from build123d import *

# Parameters (mm, degrees)
SKETCH1_W           = 6
SKETCH1_H           = 4
BOSS_EXTRUDE1_DEPTH = 3


with BuildPart() as part:
    # Sketch1 → Boss-Extrude1 (new body)
    with BuildSketch(Plane.XY):
        Polygon((0, 29.9), (5, 29.9), (5, 32.9), (20.8, 32.9), (20.8, 29.9), (33, 29.9), (33, 32.9), (48.8, 32.9), (48.8, 29.9), (53.8, 29.9), (53.8, 22.85), (56.9, 22.85), (56.9, 7.05), (53.8, 7.05), (53.8, 0), (48.8, 0), (48.8, -3.1), (33, -3.1), (33, 0), (20.8, 0), (20.8, -3.1), (5, -3.1), (5, 0), (0, 0), (0, 7.05), (-3.1, 7.05), (-3.1, 22.85), (0, 22.85), align=None)
        with Locations((33.8, 12)):
            Rectangle(SKETCH1_W, SKETCH1_H, mode=Mode.SUBTRACT)
    extrude(amount=BOSS_EXTRUDE1_DEPTH)


solid = part.part
Geometry check sheet. Reference: the model listing, model coordinates, mm. A direction names the side the tool comes from. Give positions to 0.01 mm unless a question says otherwise; leave off trailing zeros. Write each loop counter-clockwise with the first axis right and the second up, starting at its lowest first coordinate (ties: lowest second). Pieces come first, ordered by that corner, then holes.
1) Release check for a two-part mould opening along Y. For faces 6 (the face through (-2, 7.05, 1)), 7 (the face through (33, 31, 1)), 8 (the face through (-2, 22.85, 1)), 9 (the face through (30.8, 12, 1)) record: released by +Y, released by -Y, zero draft, split by the parting line, or undercut.
Values follow:
face 6: released by -Y
face 7: zero draft
face 8: released by +Y
face 9: undercut
2) Cross-section at D-D (x = 29.5). Record the boundary of the cut face in (y, z).
Values follow:
outline: (0, 0) - (29.9, 0) - (29.9, 3) - (0, 3) - close
3) Thickness scan on line 1 (X direction, y = 27, z = 1); line 2 (Y direction, x = 25.5, z = 2.45). Record the ranges inside material, lowest first.
Values follow:
line 1: x = 0 to 53.8
line 2: y = 0 to 29.9
4) Go/stop test with flat-tipped pins: pin 1 Ø0.9 at (y, z) = (26.5, 1) entering from +X; pin 2 Ø1.5 at (x, z) = (51, 1.5) entering from -Y; pin 3 Ø0.9 at (x, z) = (56, 2) entering from +Y; pin 4 Ø1 at (x, y) = (11, 9) entering from -Z. Record where each tip stops, or that it passes through.
Values follow:
pin 1: stops at x = 53.8
pin 2: stops at y = 0
pin 3: stops at y = 22.85
pin 4: stops at z = 0
5) Cross-section at A-A (y = 12). Record the boundary of the cut face in (x, z), plus the area to 3 significant figures.
Values follow:
outline: (-3.1, 0) - (30.8, 0) - (30.8, 3) - (-3.1, 3) - close; (36.8, 0) - (56.9, 0) - (56.9, 3) - (36.8, 3) - close
area: 162 mm2
6) Set-up check for faces 1 (the face through (5, 31, 1)), 2 (the face through (20.8, 31, 1)), 3 (the face through (51, 29.9, 1)), 4 (the face through (53.8, 4, 1)), 5 (the face through (5, -2, 1)): record each of +Z, -Z, +X, -X, +Y, -Y from which the full face is reachable in a straight line by a thin tool's end or side.
Values follow:
face 1: +Z, -Z, -X, +Y
face 2: +Z, -Z, +Y
face 3: +Z, -Z, +X, +Y
face 4: +Z, -Z, +X, -Y
face 5: +Z, -Z, -X, -Y
7) Cross-section at C-C (y = 28.5). Record the boundary of the cut face in (x, z), plus the area to 3 significant figures.
Values follow:
outline: (0, 0) - (53.8, 0) - (53.8, 3) - (0, 3) - close
area: 161 mm2
